```python
from build123d import *

# Parameters (mm, degrees)
BOSS_EXTRUDE1_DEPTH = 8
SKETCH2_W           = 30.471838297
SKETCH2_H           = 7.887355033
BOSS_EXTRUDE2_DEPTH = 13


with BuildPart() as part:
    # Sketch1 → Boss-Extrude1 (new body)
    with BuildSketch(Plane(origin=(0, 0, 0), x_dir=(1, 0, 0), z_dir=(0, 1, 0))):
        with BuildLine():
            Line((5.74475938, 41.611912647), (-46.770116697, 41.611912647))
            Line((-46.770116697, 41.611912647), (-46.770116697, 36.54735623))
            ThreePointArc((-46.770116697, 36.54735623), (-44.629147114, 34.406386647), (-46.770116697, 32.265417064))
            Line((-46.770116697, 32.265417064), (-46.770116697, 29.455346126))
            ThreePointArc((-46.770116697, 29.455346126), (-44.629147114, 27.314376543), (-46.770116697, 25.173406959))
            Line((-46.770116697, 25.173406959), (-46.770116697, 22.138808466))
            ThreePointArc((-46.770116697, 22.138808466), (-44.629147114, 19.997838883), (-46.770116697, 17.8568693))
            Line((-46.770116697, 17.8568693), (-46.770116697, 14.877282368))
            ThreePointArc((-46.770116697, 14.877282368), (-44.629147114, 12.736312785), (-46.770116697, 10.595343202))
            Line((-46.770116697, 10.595343202), (-46.770116697, 8.20529307))
            ThreePointArc((-46.770116697, 8.20529307), (-44.629147114, 6.064323487), (-46.770116697, 3.923353904))
            Line((-46.770116697, 3.923353904), (-46.770116697, -45.574951946))
            Line((-46.770116697, -45.574951946), (5.74475938, -45.574951946))
            Line((5.74475938, -45.574951946), (5.74475938, 3.923353904))
            ThreePointArc((5.74475938, 3.923353904), (3.603789797, 6.064323487), (5.74475938, 8.20529307))
            Line((5.74475938, 8.20529307), (5.74475938, 10.595343202))
            ThreePointArc((5.74475938, 10.595343202), (3.603789797, 12.736312785), (5.74475938, 14.877282368))
            Line((5.74475938, 14.877282368), (5.74475938, 17.8568693))
            ThreePointArc((5.74475938, 17.8568693), (3.603789797, 19.997838883), (5.74475938, 22.138808466))
            Line((5.74475938, 22.138808466), (5.74475938, 25.173406959))
            ThreePointArc((5.74475938, 25.173406959), (3.603789797, 27.314376543), (5.74475938, 29.455346126))
            Line((5.74475938, 29.455346126), (5.74475938, 32.265417064))
            ThreePointArc((5.74475938, 32.265417064), (3.603789797, 34.406386647), (5.74475938, 36.54735623))
            Line((5.74475938, 36.54735623), (5.74475938, 41.611912647))
        make_face()
    extrude(amount=BOSS_EXTRUDE1_DEPTH)

    # Sketch2 → Boss-Extrude2 (add)
    with BuildSketch(Plane(origin=(0, 0, 0), x_dir=(1, 0, 0), z_dir=(0, 1, 0))):
        Polygon((-36.740368518, -19.565642265), (-4.284988799, -19.565642265), (0, -26.156147295), (0, 36.942692964), (-41.025357317, 36.942692964), (-41.025357317, -26.156147295), align=None)
        with Locations((-20.512678659, 27.89543278)):
            Rectangle(SKETCH2_W, SKETCH2_H, mode=Mode.SUBTRACT)
    extrude(amount=BOSS_EXTRUDE2_DEPTH)


solid = part.part
```
Work out the finished part from the listing and answer in its coordinate system (mm). A direction names the side the tool comes from. Give positions to 0.01 mm unless a question says otherwise; leave off trailing zeros. Order: outer loops, then holes, each group sorted by start corner. A loop starts at its lowest first (then second) coordinate and runs counter-clockwise, first axis right, second up. Notation, with made-up numbers: (12.5, 49) -> (70.5, 49) arc R23 ccw to (70.5, 73) -> close; hole circle Ø2 at (42.25, 28.25). An arc over 180 degrees is marked (long way). Answer as CSV lines item,"result". Start each with the question number.
(1) Section A-A, the plane y = 10.5 is taken. Write down the section's boundary in (x, z).
(2) For a pull along X with two mould halves and no side action, classify faces 4 (the flat face through (-21, 8, -28)), 5 (the flat face through (-46.77, 4, 20)), 6 (the flat face through (-5.277, 10, -28)), 7 (the flat face through (-21, 4, 45.575)) as released by +X, released by -X, zero draft, split by the parting line, or undercut.
(3) Section D-D, the plane y = 1.5 is taken. Write down the section's boundary in (x, z), plus the area to 3 significant figures.
(4) Each of these flat-tipped pins is pushed along its axis until it touches: pin 1 Ø1 at (x, y) = (-15, 9.5) entering from -Z; pin 2 Ø1.5 at (x, y) = (-19, 11) entering from +Z; pin 3 Ø2.5 at (y, z) = (10, 2.5) entering from +X. Where does it stop, or does it pass through?
(5) Section C-C, the plane z = 3.5 is taken. Write down the section's boundary in (x, y), plus the area to 3 significant figures.
(6) Section B-B, the plane x = -21 is taken. Write down the section's boundary in (y, z).
(7) Which of the six approach directions +Z, -Z, +X, -X, +Y, -Y give full straight-line access (tool end or side, diameter ignored) to faces 1 (the flat face through (-20, 10, -36.943)), 2 (the flat face through (-35.749, 10, -28)), 3 (the flat face through (-21, 10, 19.566))?
(8) Consider line 1 along Z through (x, y) = (-32.5, 9.25); line 2 along X through (y, z) = (9, -29.5); line 3 along X through (y, z) = (10.75, 9). Determine where each line is inside the solid, lowest interval first.
Entries:
1,outline,"(-41.03, -36.94) -> (0, -36.94) -> (0, 26.16) -> (-4.28, 19.57) -> (-36.74, 19.57) -> (-41.03, 26.16) -> close; hole (-35.75, -31.84) -> (-5.28, -31.84) -> (-5.28, -23.95) -> (-35.75, -23.95) -> close"
2,face 4,"undercut"
2,face 5,"released by -X"
2,face 6,"undercut"
2,face 7,"zero draft"
3,outline,"(-46.77, -41.61) -> (5.74, -41.61) -> (5.74, -36.55) arc R2.14 cw to (5.74, -32.27) -> (5.74, -29.46) arc R2.14 cw to (5.74, -25.17) -> (5.74, -22.14) arc R2.14 cw to (5.74, -17.86) -> (5.74, -14.88) arc R2.14 cw to (5.74, -10.6) -> (5.74, -8.21) arc R2.14 cw to (5.74, -3.92) -> (5.74, 45.57) -> (-46.77, 45.57) -> (-46.77, -3.92) arc R2.14 cw to (-46.77, -8.21) -> (-46.77, -10.6) arc R2.14 cw to (-46.77, -14.88) -> (-46.77, -17.86) arc R2.14 cw to (-46.77, -22.14) -> (-46.77, -25.17) arc R2.14 cw to (-46.77, -29.46) -> (-46.77, -32.27) arc R2.14 cw to (-46.77, -36.55) -> close"
3,area,"4,510 mm²"
4,pin 1,"z = -36.94"
4,pin 2,"z = 19.57"
4,pin 3,"x = 0"
5,outline,"(-46.77, 0) -> (5.74, 0) -> (5.74, 8) -> (0, 8) -> (0, 13) -> (-41.03, 13) -> (-41.03, 8) -> (-46.77, 8) -> close"
5,area,"625 mm²"
6,outline,"(0, -41.61) -> (8, -41.61) -> (8, -36.94) -> (13, -36.94) -> (13, -31.84) -> (8, -31.84) -> (8, -23.95) -> (13, -23.95) -> (13, 19.57) -> (8, 19.57) -> (8, 45.57) -> (0, 45.57) -> close"
7,face 1,"-Z, +X, -X, +Y"
7,face 2,"+Y"
7,face 3,"+Z, +Y"
8,line 1,"-36.94 to -31.84, -23.95 to 19.57"
8,line 2,"-41.03 to -35.75, -5.28 to 0"
8,line 3,"-41.03 to 0"
